Could you check a few things on this model? Use its own coordinates, in mm. Face numbers are marked on the shaded views. A direction names the side the tool comes from. Round coordinates to 2 decimals unless told otherwise and drop trailing zeros. Loops run counter-clockwise (first coordinate to the right, second up) from the corner with the lowest first, then second, coordinate; pieces in that order, holes last. Notation, with made-up numbers: (-30.75, 29) -> (1.25, 29) arc R27 cw to (1.25, 58) -> close; hole circle Ø3 at (24, 4). An arc over 180 degrees is marked (long way). Write each question's results on one line, items separated by ' | '.
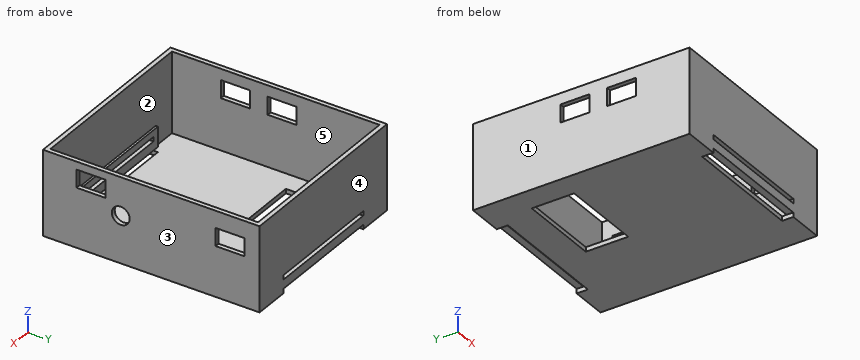
Autodesk Inventor part; units mm, degrees
ref_plane "YZ Plane" through (0, 0, 0) normal (1, 0, 0) x (0, 1, 0)
ref_plane "XZ Plane" through (0, 0, 0) normal (0, 1, 0) x (-1, 0, 0)
ref_plane "XY Plane" through (0, 0, 0) normal (0, 0, 1) x (1, 0, 0)
sketch "Sketch1" plane through (0, 0, 0) normal (0, 0, 1) x (1, 0, 0)
  line L0 (-41, -46.5) -> (41, -46.5)
  line L1 (41, -46.5) -> (41, 46.5)
  line L2 (41, 46.5) -> (-41, 46.5)
  line L3 (-41, 46.5) -> (-41, -46.5)
  line L4 (-41, -46.5) -> (41, 46.5) construction
  line L5 (41, -46.5) -> (-41, 46.5) construction
  line L6 (43, 48.5) -> (43, -48.5)
  line L7 (43, -48.5) -> (-43, -48.5)
  line L8 (-43, -48.5) -> (-43, 48.5)
  line L9 (-43, 48.5) -> (43, 48.5)
  point P0 (0, 0)
  dimension "d0" = 93
  dimension "d1" = 82
  dimension "d2" = 2
extrude "Extrusion1" add sketch "Sketch1" along normal blind 40
sketch "Sketch2" plane through (0, 0, 0) normal (0, 0, -1) x (-1, 0, 0)
  line L0 (41, 46.5) -> (41, -46.5)
  line L1 (41, -46.5) -> (-41, -46.5)
  line L2 (-41, -46.5) -> (-41, 46.5)
  line L3 (-41, 46.5) -> (41, 46.5)
  line L4 (-43, 48.5) -> (-43, -48.5)
  line L5 (-43, -48.5) -> (43, -48.5)
  line L6 (43, -48.5) -> (43, 48.5)
  line L7 (43, 48.5) -> (-43, 48.5)
  point P0 (0, 0)
extrude "Extrusion2" add sketch "Sketch2" along normal blind 2 contours L0 L1 L2 L3 | L7 L6 L5 L4
sketch "Sketch4" plane through (0, 0, -2) normal (0, 0, -1) x (-1, 0, 0)
  line L0 (41, 46.5) -> (41, -46.5)
  line L1 (-41, 46.5) -> (41, 46.5)
  line L2 (-41, -46.5) -> (-41, 46.5)
  line L3 (41, -46.5) -> (-41, -46.5)
  line L4 (0, 46.5) -> (0, 31.5)
  line L5 (41, -46.5) -> (41, 46.5)
  line L6 (41, 31.5) -> (37, 31.5)
  line L7 (-41, 46.5) -> (-41, -46.5)
  line L8 (-41, 16) -> (-7, 16)
  line L9 (23, -46.5) -> (23, 3.5)
  line L10 (37, 31.5) -> (-10, 31.5)
  line L11 (-10, 31.5) -> (-10, 3.5)
  line L12 (-10, 3.5) -> (37, 3.5)
  line L13 (37, 3.5) -> (37, 31.5)
  point P0 (0, 0)
  dimension "d11" = 15
  dimension "d12" = 4
  dimension "d13" = 34
  dimension "d14" = 50
extrude "Extrusion4" cut sketch "Sketch4" against normal blind 2 contours L13 L12 L11 L10
sketch "Sketch8" plane through (-43, 48.5, 40) normal (0, 1, 0) x (1, 0, 0)
  line L0 (0, 0) -> (0, 42)
  line L1 (86, 0) -> (0, 0)
  line L2 (86, 42) -> (86, 0)
  line L3 (0, 42) -> (86, 42)
  line L4 (6, 42) -> (53, 42)
  line L5 (43, 42) -> (16, 42)
  line L6 (43, 42) -> (43, 40)
  line L7 (43, 40) -> (43, 36)
  line L8 (43, 36) -> (43, 34)
  line L9 (84, 40) -> (2, 40)
  line L10 (16, 42) -> (70, 42)
  line L11 (70, 42) -> (70, 40)
  line L12 (70, 40) -> (16, 40)
  line L13 (16, 40) -> (16, 42)
  line L14 (16, 34) -> (70, 34)
  line L15 (70, 34) -> (70, 36)
  line L16 (70, 36) -> (16, 36)
  line L17 (16, 36) -> (16, 34)
  dimension "d29" = 27
  dimension "d30" = 2
  dimension "d31" = 4
  dimension "d32" = 2
  dimension "d33" = 54
sketch "Sketch9" plane through (-43, 48.5, 40) normal (0, 1, 0) x (1, 0, 0)
  line L0 (70, 42) -> (73, 42)
  line L1 (6, 42) -> (53, 42)
  line L2 (16, 42) -> (13, 42)
  line L3 (70, 34) -> (70, 31)
  line L4 (73, 42) -> (13, 42)
  line L5 (13, 42) -> (13, 31)
  line L6 (13, 31) -> (73, 31)
  line L7 (73, 31) -> (73, 42)
  point P0 (43, 40)
  dimension "d34" = 3
  dimension "d35" = 3
  dimension "d36" = 3
extrude "Extrusion8" add sketch "Sketch9" against normal blind 3
extrude "Extrusion9" cut sketch "Sketch8" against normal blind 5 contours L16 L15 L14 L8 | L8 L14 L17 L16 | L3 L6 L9 L13 | L11 L9 L6 L3
sketch "Sketch10" plane through (0, 0, 40) normal (0, 0, 1) x (1, 0, 0)
  line L0 (-41, -46.5) -> (-41, 46.5)
  line L1 (-41, 46.5) -> (41, 46.5)
  line L2 (41, 46.5) -> (41, -46.5)
  line L3 (41, -46.5) -> (-41, -46.5)
  line L4 (43, -48.5) -> (43, 48.5)
  line L5 (43, 48.5) -> (-43, 48.5)
  line L6 (-43, 48.5) -> (-43, -48.5)
  line L7 (-43, -48.5) -> (43, -48.5)
  point P0 (0, 0)
extrude "Extrusion10" cut sketch "Sketch10" against normal blind 4
sketch "Sketch11" plane through (-43, -48.5, -2) normal (-1, 0, 0) x (0, 0, 1)
  line L0 (2, 95) -> (38, 95)
  line L1 (2, 95) -> (2, 2)
  line L2 (11, 95) -> (2, 95)
  line L3 (2, 95) -> (2, 62.2)
  line L4 (2, 80) -> (2, 52)
  line L5 (2, 62.2) -> (21, 62.2)
  circle A0 centre (21, 62.2) radius 4
  line L6 (2, 79) -> (30.5, 79)
  line L7 (30.5, 95) -> (30.5, 83)
  line L8 (30.5, 83) -> (30.5, 72)
  line L9 (30.5, 79) -> (30.5, 72)
  line L10 (26.5, 82) -> (34.5, 82)
  line L11 (34.5, 82) -> (34.5, 69)
  line L12 (34.5, 69) -> (26.5, 69)
  line L13 (26.5, 69) -> (26.5, 82)
  line L14 (26.5, 82) -> (34.5, 69) construction
  line L15 (34.5, 82) -> (26.5, 69) construction
  line L16 (2, 7) -> (26.5, 7)
  line L17 (2, 2) -> (38, 2)
  line L18 (26.42, 2) -> (26.42, 13.2)
  line L19 (22.42, 6.7) -> (22.42, 19.7)
  line L20 (22.42, 19.7) -> (30.42, 19.7)
  line L21 (30.42, 19.7) -> (30.42, 6.7)
  line L22 (30.42, 6.7) -> (22.42, 6.7)
  line L23 (22.42, 6.7) -> (30.42, 19.7) construction
  line L24 (22.42, 19.7) -> (30.42, 6.7) construction
  line L25 (2, 2) -> (38, 2)
  line L26 (2, 95) -> (2, 2)
  line L27 (2, 2) -> (2, 48.5)
  line L28 (2, 2) -> (2, 95)
  line L29 (28, 48.5) -> (2, 48.5)
  circle A1 centre (21, 34.8) radius 4
  line L30 (26.5, 15) -> (34.5, 15)
  line L31 (34.5, 15) -> (34.5, 28)
  line L32 (34.5, 28) -> (26.5, 28)
  line L33 (26.5, 28) -> (26.5, 15)
  line L34 (22.42, 90.3) -> (22.42, 77.3)
  line L35 (22.42, 77.3) -> (30.42, 77.3)
  line L36 (30.42, 77.3) -> (30.42, 90.3)
  line L37 (30.42, 90.3) -> (22.42, 90.3)
  point P0 (30.5, 75.5)
  dimension "d43" = 32.8
  dimension "d44" = 19
  dimension "d45" = 8
  dimension "d48" = 28.5
  dimension "d50" = 12
  dimension "d51" = 11
  dimension "d52" = 8
  dimension "d53" = 13
  dimension "d54" = 24.5
  dimension "d55" = 11.2
  dimension "d56" = 13
  dimension "d57" = 8
extrude "Extrusion11" cut sketch "Sketch11" against normal through all contours L34 L37 L36 L10 L13 L6 | L6 L13 L35 L34 | L13 L10 L36 L6 | L6 L36 L35 L13 | L33 L32 L31 L30 L21 L20 | L20 L21 L30 L33 | A1
sketch "Sketch12" plane through (-43, -48.5, -2) normal (-1, 0, 0) x (0, 0, 1)
  line L0 (38, 0) -> (38, 97)
  line L1 (38, 97) -> (0, 97)
  line L2 (0, 0) -> (0, 97)
  line L3 (38, 0) -> (0, 0)
  point P0 (2, 48.5)
extrude "Extrusion12" add sketch "Sketch12" against normal up to surface (2 mm away)
sketch "Sketch13" plane through (-43, -48.5, -2) normal (-1, 0, 0) x (0, 0, 1)
  line L0 (38, 0) -> (38, 97)
  line L1 (38, 97) -> (0, 97)
  line L2 (38, 0) -> (0, 0)
  line L3 (2, 95) -> (38, 95)
  line L4 (2, 95) -> (2, 2)
  line L5 (2, 2) -> (38, 2)
  line L6 (2, 72) -> (29, 72)
  line L7 (29.0235, 95) -> (29.0235, 51.4)
  line L8 (25.0235, 57.9) -> (33.0235, 57.9)
  line L9 (33.0235, 57.9) -> (33.0235, 44.9)
  line L10 (33.0235, 44.9) -> (25.0235, 44.9)
  line L11 (25.0235, 44.9) -> (25.0235, 57.9)
  line L12 (25.0235, 57.9) -> (33.0235, 44.9) construction
  line L13 (33.0235, 57.9) -> (25.0235, 44.9) construction
  line L14 (29.0235, 51.4) -> (29.0235, 30.4)
  line L15 (25.0235, 36.9) -> (33.0235, 36.9)
  line L16 (33.0235, 36.9) -> (33.0235, 23.9)
  line L17 (33.0235, 23.9) -> (25.0235, 23.9)
  line L18 (25.0235, 23.9) -> (25.0235, 36.9)
  line L19 (25.0235, 36.9) -> (33.0235, 23.9) construction
  line L20 (33.0235, 36.9) -> (25.0235, 23.9) construction
  line L21 (0, 0) -> (0, 97)
  point P0 (2, 48.5)
  dimension "d60" = 27
  dimension "d61" = 43.6
  dimension "d62" = 8
  dimension "d63" = 13
  dimension "d64" = 21
  dimension "d65" = 8
  dimension "d66" = 13
extrude "Extrusion13" cut sketch "Sketch13" against normal blind 8 contours L15 L16 L17 L18 | L8 L9 L10 L14 L7 | L7 L14 L10 L11 L8
mirror "Mirror3" about plane through (0, 0, 0) normal (0, 1, 0) of "Extrusion8", "Extrusion9"
sketch "Sketch14" plane through (0, 0, -2) normal (0, 0, -1) x (-1, 0, 0)
  line L0 (-27, -48.5) -> (-27, -43.5)
  line L1 (-27, -43.5) -> (27, -43.5)
  line L2 (27, -43.5) -> (27, -48.5)
  line L3 (27, -48.5) -> (43, -48.5)
  line L4 (43, -48.5) -> (43, 48.5)
  line L5 (43, 48.5) -> (27, 48.5)
  line L6 (27, 48.5) -> (27, 43.5)
  line L7 (27, 43.5) -> (-27, 43.5)
  line L8 (-27, 43.5) -> (-27, 48.5)
  line L9 (-27, 48.5) -> (-43, 48.5)
  line L10 (-43, 48.5) -> (-43, -48.5)
  line L11 (-43, -48.5) -> (-27, -48.5)
  line L12 (-41, -46.5) -> (-41, 46.5)
  line L13 (-41, 46.5) -> (-30, 46.5)
  line L14 (30, 46.5) -> (41, 46.5)
  line L15 (-30, 46.5) -> (-30, 45.5)
  line L16 (-4.5, 29.5) -> (32, 29.5)
  line L17 (32, 29.5) -> (32, 10.5)
  line L18 (32, 10.5) -> (-4.5, 10.5)
  line L19 (-4.5, 10.5) -> (-4.5, 29.5)
  line L20 (-10, 3.5) -> (-10, 31.5)
  line L21 (-10, 31.5) -> (37, 31.5)
  line L22 (37, 31.5) -> (37, 3.5)
  line L23 (37, 3.5) -> (-10, 3.5)
extrude "Extrusion14" add sketch "Sketch14" against normal up to surface (2 mm away) contours L20 L21 L22 L23
properties part number "chest_piece_bottom_2"
1) I want a section at A-A, the plane x = -1.5. Write out the boundary of the cut face in (y, z), plus the area to 3 significant figures.
Model answer:
outline: (-48.5, 0) -> (-45.5, 0) -> (-45.5, 4) -> (-48.5, 4) -> close; (-48.5, 6) -> (-45.5, 6) -> (-45.5, 9) -> (-46.5, 9) -> (-46.5, 36) -> (-48.5, 36) -> close; (-43.5, -2) -> (10.5, -2) -> (10.5, 0) -> (-43.5, 0) -> close; (29.5, -2) -> (43.5, -2) -> (43.5, 0) -> (29.5, 0) -> close; (45.5, 0) -> (48.5, 0) -> (48.5, 4) -> (45.5, 4) -> close; (45.5, 6) -> (48.5, 6) -> (48.5, 36) -> (46.5, 36) -> (46.5, 9) -> (45.5, 9) -> close | area: 286 mm2
2) I need wall thicknesses on line 1 (X direction, y = -37.5, z = 6.5); line 2 (Y direction, x = 37.5, z = 1.5); line 3 (Y direction, x = 41.6, z = 19). Which ranges of each line are inside material? Lowest first, please.
Model answer:
line 1: x = -43 to -41, 41 to 43 | line 2: y = -48.5 to -46.5, 46.5 to 48.5 | line 3: y = -48.5 to -17.7, -9.7 to 48.5
3) I want a section at D-D, the plane x = 18.5. Write out the boundary of the cut face in (y, z), plus the area to 3 significant figures.
Model answer:
outline: (-48.5, 0) -> (-45.5, 0) -> (-45.5, 4) -> (-48.5, 4) -> close; (-48.5, 6) -> (-45.5, 6) -> (-45.5, 9) -> (-46.5, 9) -> (-46.5, 36) -> (-48.5, 36) -> close; (-43.5, -2) -> (43.5, -2) -> (43.5, 0) -> (-43.5, 0) -> close; (45.5, 0) -> (48.5, 0) -> (48.5, 4) -> (45.5, 4) -> close; (45.5, 6) -> (48.5, 6) -> (48.5, 36) -> (46.5, 36) -> (46.5, 9) -> (45.5, 9) -> close | area: 324 mm2
4) If we mould it in two halves opening along X, with no side actions, what happens to the marked faces 1, 2 and 3? For each: released by +X, released by -X, zero draft, split by the parting line, or undercut.
Model answer:
face 1: released by -X | face 2: undercut | face 3: released by +X
5) For the marked faces 4 and 5, which set-ups out of +Z, -Z, +X, -X, +Y, -Y let a thin tool reach every point of the face, with its end or its side?
Model answer:
face 4: +Z, -Z, +X, -X, +Y | face 5: +Z
6) I want a section at C-C, the plane z = 19. Write out the boundary of the cut face in (x, y).
Model answer:
outline: (-43, -48.5) -> (43, -48.5) -> (43, -17.7) -> (41, -17.7) -> (41, -46.5) -> (-41, -46.5) -> (-41, 46.5) -> (41, 46.5) -> (41, -9.7) -> (43, -9.7) -> (43, 48.5) -> (-43, 48.5) -> close
7) I'm going to push flat-ended pins straight in: pin 1 (4 mm diameter, centred on x = -4, y = -27, fed in from +Z); pin 2 (2.5 mm diameter, centred on x = -2.5, y = -47, fed in from -Z). Where does each tip first touch, or does it pass through?
Model answer:
pin 1: stops at z = 0 | pin 2: stops at z = 0
8) I want a section at B-B, the plane y = -13.7. Write out the boundary of the cut face in (x, z).
Model answer:
outline: (-43, -2) -> (43, -2) -> (43, 15) -> (41, 15) -> (41, 0) -> (-41, 0) -> (-41, 23.02) -> (-43, 23.02) -> close; (-43, 31.02) -> (-41, 31.02) -> (-41, 36) -> (-43, 36) -> close; (41, 23) -> (43, 23) -> (43, 36) -> (41, 36) -> close
